Here's how the part is built. I have some questions about the finished solid (model axes, mm). Face numbers are marked on the shaded views. A direction names the side the tool comes from. Coordinates: 2 decimals unless noted, no trailing zeros. Loops run counter-clockwise (first coordinate to the right, second up) from the corner with the lowest first, then second, coordinate; pieces in that order, holes last. Notation, with made-up numbers: M 30,48.5 L 59,48.5 A23 ccw 59,77.5 Z; hole C -40,15 d11. An arc over 180 degrees is marked long. Use one line per item in the form item = value. Start each with the question number.
(1) Will these pins go through, and if not, where does the flat tip stop? P1, Ø4.5, axis at x = -11, y = -1.5, coming from the -Z side; P2, Ø2.5, axis at x = 0, z = -6.1, coming from the -Y side; P3, Ø1.5, axis at y = 0, z = -6.5, coming from the +X side.
(2) Imagine slicing it at A-A, the plane x = 0. Please give me the cut outline in (y, z), and give its area (3 significant figures).
(3) Imagine slicing it at C-C, the plane y = 10. Please give me the cut outline in (x, z), and give its area (3 significant figures).
(4) Imagine slicing it at B-B, the plane x = 7.5. Please give me the cut outline in (y, z).
(5) On a 3-axis mill with a long thin cutter (end or side, diameter ignored), from which of +Z, -Z, +X, -X, +Y, -Y can I reach the whole of each face in a straight line? I mean the marked faces 1 and 2. Say none if no direction works.
(6) Please list where these lines run through material, in increasing order: L1, parallel to Z at x = 0, y = 0.85; L2, parallel to Z at x = -21, y = 1.25; L3, parallel to X at y = 13.5, z = -4.
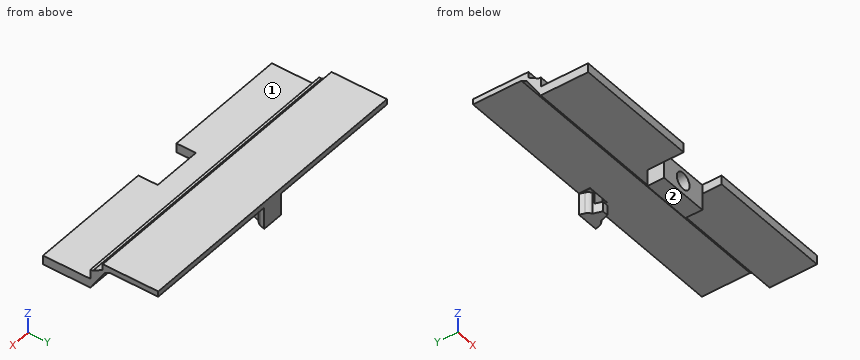
```python
from build123d import *

# Parameters (mm, degrees)
EXTRUDE_1_DEPTH     = 27
SKETCH_2_W          = 9
SKETCH_2_H          = 4
CUT_EXTRUDE_1_DEPTH = 4
SKETCH_3_W          = 9
SKETCH_3_H          = 3.038101075
EXTRUDE_2_DEPTH     = 3
SKETCH_4_R          = 1.5
CUT_EXTRUDE_2_DEPTH = 9
EXTRUDE_3_DEPTH     = 2
CUT_EXTRUDE_8_DEPTH = 3.9


with BuildPart() as part:
    # 草图1 → 凸台-拉伸1 (new, symmetric)
    with BuildSketch(Plane(origin=(0, 0, 0), x_dir=(0, 0, -1), z_dir=(1, 0, 0))):
        Polygon((5.5, -5.234874936), (5.5, -1.276151444), (5.5, 1.303226139), (5.5, 3.316049082), (1.495683541, 5.841749257), (0.996390194, 6.822725158), (0.996390194, 8.881545648), (0.996390194, 13.350016649), (0.996390194, 15.531060696), (0, 15.531060696), (0, 13.265125064), (0, 9.02431695), (0, 5.531060696), (1.075983727, 5.531060696), (2.127060271, 3.7449116), (2.127060271, 3.316049082), (3.852001832, 3.316049082), (3.852001832, -5.234874936), align=None)
    extrude(amount=EXTRUDE_1_DEPTH, both=True)

    # 草图2 → 切除-拉伸1 (cut)
    with BuildSketch(Plane(origin=(0, 0, -5.5), x_dir=(-1, 0, 0), z_dir=(0, 0, -1))):
        with Locations((0, -3.734874936)):
            Rectangle(SKETCH_2_W, SKETCH_2_H)
    extrude(amount=-CUT_EXTRUDE_1_DEPTH, mode=Mode.SUBTRACT)

    # 草图3 → 凸台-拉伸2 (add)
    with BuildSketch(Plane(origin=(0, 0, -5.5), x_dir=(-1, 0, 0), z_dir=(0, 0, -1))):
        with Locations((0, -0.215824399)):
            Rectangle(SKETCH_3_W, SKETCH_3_H)
    extrude(amount=EXTRUDE_2_DEPTH)

    # 草图4 → 切除-拉伸2 (cut)
    with BuildSketch(Plane.XZ.offset(1.734874936)):
        with Locations(Location((0, -6.102001832, 0), (0, 0, 270))):
            Circle(SKETCH_4_R)
    extrude(amount=-CUT_EXTRUDE_2_DEPTH, mode=Mode.SUBTRACT)

    # 草图6 → 凸台-拉伸3 (add, symmetric)
    with BuildSketch(Plane(origin=(0, 0, 0), x_dir=(0, 0, -1), z_dir=(1, 0, 0))):
        Polygon((0.975132856, 15.531060696), (4.975132856, 15.531060696), (4.975132856, 12.331060696), (3.175132856, 12.331060696), (3.175132856, 13.531060696), (2.0593477, 13.531060696), (0.975132856, 13.531060696), align=None)
    extrude(amount=EXTRUDE_3_DEPTH, both=True)

    # 草图7 → 切除-拉伸8 (cut)
    with BuildSketch(Plane(origin=(0, 0, -4.975132856), x_dir=(-1, 0, 0), z_dir=(0, 0, -1))):
        with BuildLine():
            Line((1, 13.831060696), (0.52341558, 12.331060696))
            Line((0.52341558, 12.331060696), (2, 12.331060696))
            Line((2, 12.331060696), (2, 15.531060696))
            Line((2, 15.531060696), (1.723060875, 14.659423543))
            ThreePointArc((1.723060875, 14.659423543), (1.447645575, 14.170073989), (1, 13.831060696))
        make_face()
        with BuildLine():
            ThreePointArc((-1.723060875, 14.659423543), (-1.447645575, 14.170073989), (-1, 13.831060696))
            Line((-1, 13.831060696), (-0.52341558, 12.331060696))
            Line((-0.52341558, 12.331060696), (-2, 12.331060696))
            Line((-2, 12.331060696), (-2, 15.531060696))
            Line((-2, 15.531060696), (-1.723060875, 14.659423543))
        make_face()
    extrude(amount=-CUT_EXTRUDE_8_DEPTH, mode=Mode.SUBTRACT)


solid = part.part
```
Answer:
q1.P1 = -5.5
q1.P2 = 12.33
q1.P3 = 4.5
q2.outline = M -1.73,-8.5 L 1.3,-8.5 L 1.3,-7.6 L -1.73,-7.6 Z; M -1.73,-4.6 L 3.88,-4.6 L 5.84,-1.5 L 6.82,-1 L 13.53,-1 L 13.53,-3.18 L 12.33,-3.18 L 12.33,-4.98 L 15.53,-4.98 L 15.53,0 L 5.53,0 L 5.53,-1.08 L 3.74,-2.13 L 3.32,-2.13 L 3.32,-3.85 L -1.73,-3.85 Z
q2.area = 31.3 mm²
q3.outline = M -27,-1 L 27,-1 L 27,0 L -27,0 Z
q3.area = 53.8 mm²
q4.outline = M -5.23,-5.5 L 3.32,-5.5 L 5.84,-1.5 L 6.82,-1 L 15.53,-1 L 15.53,0 L 5.53,0 L 5.53,-1.08 L 3.74,-2.13 L 3.32,-2.13 L 3.32,-3.85 L -5.23,-3.85 Z
q5.face_1 = +Z, +X, -X, -Y
q5.face_2 = -Z, +X, -X, +Y, -Y
q6.L1 = -8.5 to -7.6, -4.6 to -3.85
q6.L2 = -5.5 to -3.85
q6.L3 = -0.89 to 0.89
